Here's how the part is built. I have some questions about the finished solid (model axes, mm). A direction names the side the tool comes from. Round coordinates to 2 decimals unless told otherwise and drop trailing zeros. Write each loop counter-clockwise with the first axis right and the second up, starting at its lowest first coordinate (ties: lowest second). Pieces come first, ordered by that corner, then holes. Notation, with made-up numbers: (19, -1.5) -> (58, -1.5) arc R17 ccw to (58, 9.5) -> close; hole circle Ø2 at (73, 68.5). An arc over 180 degrees is marked (long way). Put each result on its own line as item: value. Start each with the question number.
1. I need wall thicknesses on probe 1 along Z at (x, y) = (-5, 11.5); probe 2 along Y at (x, z) = (-40, 37); probe 3 along X at (y, z) = (-17.5, 7). Which ranges of each line are inside material? Lowest first, please. Write a range as from..to.
2. Which directions (+Z, -Z, +X, -X, +Y, -Y) give clear straight access to the entire face, cutting with the end or side of a thin tool? Please do faces 1 (the face through (-28, -28, 44)), 2 (the face through (-12, -21, 40)).
3. Suppose I cut it at D-D (y = -48.5). Please give me the cut outline in (x, z), then the cut area to 3 significant figures.
4. Suppose I cut it at B-B (x = -39.5). Please give me the cut outline in (y, z).
5. Suppose I cut it at C-C (z = 27). Please give me the cut outline in (x, y).
6. Suppose I cut it at A-A (y = 0). Please give me the cut outline in (x, z), then the cut area to 3 significant figures.
7. For pin 1 (10 mm diameter, centred on x = -41.5, y = -47.5, fed in from +Z); pin 2 (3 mm diameter, centred on x = -35.5, y = -29, fed in from -Z), each with a flat end and sliding along its axis, tell me the tip position at first contact or that it passes through.
```python
from build123d import *

# Parameters (mm, degrees)
F0_W     = 81.4292449504
F0_H     = 93.3251976967
F1_DEPTH = 40
F2_R     = 29.0333900914
F3_DEPTH = 50
F4_R     = 31.3063799937
F4_R_2   = 29.0333900914
F5_DEPTH = 4


with BuildPart() as f1:
    # F0 (on Top) → F1 (new body)
    with BuildSketch(Plane.XY):
        with Locations((-29.1790282354, -11.1290290952)):
            Rectangle(F0_W, F0_H)
    extrude(amount=F1_DEPTH)

    # F2 (on face) → F3 (cut)
    with BuildSketch(Plane.XY.offset(40)):
        with Locations((-36.7132276297, 0)):
            Circle(F2_R)
    extrude(amount=-F3_DEPTH, mode=Mode.SUBTRACT)

    # F4 (on face) → F5 (join)
    with BuildSketch(Plane.XY.offset(40)):
        with Locations((-36.7132276297, 0)):
            Circle(F4_R)
        with Locations((-36.7132276297, 0)):
            Circle(F4_R_2, mode=Mode.SUBTRACT)
    extrude(amount=F5_DEPTH)


solid = f1.part
```
Verdict:
1. probe 1: z = 0..40
1. probe 2: y = -57.79..-28.85, 28.85..35.53
1. probe 3: x = -69.89..-59.88, -13.55..11.54
2. face 1: +Z, +X, -X, +Y, -Y
2. face 2: +Z
3. outline: (-69.89, 0) -> (11.54, 0) -> (11.54, 40) -> (-69.89, 40) -> close
3. area: 3,260 mm^2
4. outline: (-57.79, 0) -> (-28.9, 0) -> (-28.9, 44) -> (-31.18, 44) -> (-31.18, 40) -> (-57.79, 40) -> close; (28.9, 0) -> (35.53, 0) -> (35.53, 40) -> (31.18, 40) -> (31.18, 44) -> (28.9, 44) -> close
5. outline: (-69.89, -57.79) -> (11.54, -57.79) -> (11.54, 35.53) -> (-69.89, 35.53) -> close; hole circle Ø58.07 at (-36.71, 0)
6. outline: (-69.89, 0) -> (-65.75, 0) -> (-65.75, 44) -> (-68.02, 44) -> (-68.02, 40) -> (-69.89, 40) -> close; (-7.68, 0) -> (11.54, 0) -> (11.54, 40) -> (-5.41, 40) -> (-5.41, 44) -> (-7.68, 44) -> close
6. area: 953 mm^2
7. pin 1: stops at z = 40
7. pin 2: stops at z = 0
